from build123d import *

# Parameters (mm, degrees)
F0_W     = 47
F0_H     = 30
F1_DEPTH = 3
F0_W_2   = 3
F2_DEPTH = 60
F4_D     = 4.5
F4_DEPTH = 12.4
F6_D     = 5.5
F6_DEPTH = 12.4
F7_SIZE  = 2


with BuildPart() as f1:
    # F0 (on Top) → F1 (new body)
    with BuildSketch(Plane.XY):
        with Locations((1.397237, -14.812001)):
            Rectangle(F0_W, F0_H)
    extrude(amount=F1_DEPTH)

    # F0 (on Top) → F2 (join)
    with BuildSketch(Plane.XY):
        with Locations((-23.602763, -14.812001)):
            Rectangle(F0_W_2, F0_H)
    extrude(amount=F2_DEPTH)

    # F4
    with Locations(Plane(origin=(-25.102763, 0, 0), x_dir=(0, -1, 0), z_dir=(-1, 0, 0))):
        with Locations((5.812001, 54.5), (23.812001, 36.5)):
            Hole(F4_D / 2, depth=F4_DEPTH)

    # F6
    with Locations(Plane.XY.offset(3)):
        with Locations((-10.102763, -14.812001), (14.897237, -14.812001)):
            Hole(F6_D / 2, depth=F6_DEPTH)

    # F7
    f7_edges = [f1.edges().sort_by_distance(p)[0] for p in [
        (-23.602763, -29.812001, 60),
        (-23.602763, 0.187999, 60),
        (24.897237, -29.812001, 1.5),
        (24.897237, 0.187999, 1.5),
    ]]
    chamfer(f7_edges, length=F7_SIZE)


solid = f1.part
Here's how the part is built. I have some questions about the finished solid (model axes, mm). A direction names the side the tool comes from. Coordinates: 2 decimals unless noted, no trailing zeros. Order: outer loops, then holes, each group sorted by start corner. A loop starts at its lowest first (then second) coordinate and runs counter-clockwise, first axis right, second up. Notation, with made-up numbers: (-37, 60) -> (-10, 60) arc R23 ccw to (-10, 69) -> close; hole circle Ø4 at (70, 69). An arc over 180 degrees is marked (long way). Answer in a Markdown table with one row per item.
(1) I want a section at C-C on x = -3. List the corners of the cut face in (y, z) for me, then the cut area to 3 significant figures.
Answer key:
| item | result |
|---|---|
| outline | (-29.81, 0) -> (0.19, 0) -> (0.19, 3) -> (-29.81, 3) -> close |
| area | 90.0 mm^2 |
(2) I want a section at D-D on z = 6.5. List the corners of the cut face in (x, y) for me, then the cut area to 3 significant figures.
Answer key:
| item | result |
|---|---|
| outline | (-25.1, -29.81) -> (-22.1, -29.81) -> (-22.1, 0.19) -> (-25.1, 0.19) -> close |
| area | 90.0 mm^2 |
(3) Will these pins go through, and if not, where does the flat tip stop? pin 1 Ø8 at (y, z) = (-18.5, 47.5) entering from +X; pin 2 Ø6.5 at (x, y) = (14.9, -14.81) entering from +Z.
Answer key:
| item | result |
|---|---|
| pin 1 | x = -22.1 |
| pin 2 | z = 3 |
(4) Please list where these lines run through material, in increasing order: probe 1 along X at (y, z) = (-24.5, 14.5); probe 2 along Z at (x, y) = (-5, -22); probe 3 along Y at (x, z) = (-23, 54).
Answer key:
| item | result |
|---|---|
| probe 1 | -25.1 to -22.1 |
| probe 2 | 0 to 3 |
| probe 3 | -29.81 to -8.01, -3.62 to 0.19 |
(5) I want a section at B-B on y = -20.5. List the corners of the cut face in (x, z) for me.
Answer key:
| item | result |
|---|---|
| outline | (-25.1, 0) -> (24.9, 0) -> (24.9, 3) -> (-22.1, 3) -> (-22.1, 60) -> (-25.1, 60) -> close |
(6) Thinking about a two-plate mould opening in Y: for faces 1 (the face through (-8.08, -12.95, 1.48)), 2 (the face through (-22.103, -15, 31)), 3 (the face through (-23.582, -22.602, 38.397)), 4 (the face through (23.911, -0.826, 1.479)), which applies, +Y half, -Y half, draft (parallel to the pull), parting line (faces both ways), or undercut?
Answer key:
| item | result |
|---|---|
| face 1 | undercut |
| face 2 | draft |
| face 3 | undercut |
| face 4 | +Y half |
(7) I want a section at A-A on z = 54.5. List the corners of the cut face in (x, y) for me, then the cut area to 3 significant figures.
Answer key:
| item | result |
|---|---|
| outline | (-25.1, -29.81) -> (-22.1, -29.81) -> (-22.1, -8.06) -> (-25.1, -8.06) -> close; (-25.1, -3.56) -> (-22.1, -3.56) -> (-22.1, 0.19) -> (-25.1, 0.19) -> close |
| area | 76.5 mm^2 |
(8) On a 3-axis mill with a long thin cutter (end or side, diameter ignored), from which of +Z, -Z, +X, -X, +Y, -Y can I reach the whole of each face in a straight line? I mean faces 5 (the face through (23.91, -28.8, 1.48)), 6 (the face through (1, -15, 3)). Say none if no direction works.
Answer key:
| item | result |
|---|---|
| face 5 | +Z, -Z, +X, -Y |
| face 6 | +Z, +X, +Y, -Y |
